Build history of the part. All positions in model axes, mm. Round coordinates to 2 decimals unless told otherwise and drop trailing zeros. Loops run counter-clockwise (first coordinate to the right, second up) from the corner with the lowest first, then second, coordinate; pieces in that order, holes last. Notation, with made-up numbers: M 9,35.5 L 28,35.5 A19 cw 28,45.5 Z; hole C 17,42.5 d11. An arc over 180 degrees is marked long. Write each question's results on one line, items separated by ' | '. Start each with the question number.
```python
from build123d import *

# Parameters (mm, degrees)
SKETCH1_R        = 7.8613
SKETCH1_R_2      = 3.93065
ROD_DEPTH        = 1228.725
HOLES_DEPTH      = 1229.77529504
HOLES_DEPTH_BACK = 1229.77529504
SKETCH3_R        = 2.1082


with BuildPart() as part:
    # Sketch1 → Rod (new body)
    with BuildSketch(Plane.XY):
        Circle(SKETCH1_R)
        Circle(SKETCH1_R_2, mode=Mode.SUBTRACT)
    extrude(amount=ROD_DEPTH)

    # Sketch3 → Holes (cut, two sides: drawn at the far end of the back side and taken through both)
    with BuildSketch(Plane(origin=(0, 0, 0), x_dir=(1, 0, 0), z_dir=(0, 1, 0)).offset(-HOLES_DEPTH_BACK)):
        with Locations(Location((0, -425.45, 0), (0, 0, 270))):
            Circle(SKETCH3_R)
        with Locations(Location((0, -666.75, 0), (0, 0, 270))):
            Circle(SKETCH3_R)
        with Locations(Location((0, -1209.675, 0), (0, 0, 270))):
            Circle(SKETCH3_R)
    extrude(amount=HOLES_DEPTH + HOLES_DEPTH_BACK, mode=Mode.SUBTRACT)


solid = part.part
```
Item 1: Drill centre lines: line 1 along Z through (x, y) = (0, -6.2) (3 decimals); line 2 along Y through (x, z) = (0.5, 783); line 3 along Y through (x, z) = (0, 854.5). Where is each one in solid material? Low to high. Write a range as [from, to].
Item 2: Drop flat-ended pins along their axis: pin 1 (5 mm diameter, centred on x = 0, z = 666.75, fed in from -Y); pin 2 (3 mm diameter, centred on x = 4, z = 363.5, fed in from -Y); pin 3 (5 mm diameter, centred on x = 3.5, z = 802.5, fed in from -Y); pin 4 (1.5 mm diameter, centred on y = -3.5, z = 394, fed in from +X). Give the stop position or say it passes through.
Item 3: Saw through at A-A, the plane z = 264. Give the cut face in (x, y), then the cut area to 3 significant figures.
Working result:
1) line 1: z = [0, 423.342], [427.558, 664.642], [668.858, 1207.567], [1211.783, 1228.725] | line 2: y = [-7.85, -3.9], [3.9, 7.85] | line 3: y = [-7.86, -3.93], [3.93, 7.86]
2) pin 1: stops at y = -7.86 | pin 2: stops at y = -7.45 | pin 3: stops at y = -7.8 | pin 4: stops at x = 7.36
3) outline: C 0,0 d15.72; hole C 0,0 d7.86 | area: 146 mm²
